Can you work these out from the model? Positions are in its coordinate system, mm. A direction names the side the tool comes from. Coordinates: 2 decimals unless noted, no trailing zeros. Order: outer loops, then holes, each group sorted by start corner. A loop starts at its lowest first (then second) coordinate and runs counter-clockwise, first axis right, second up.
```python
from build123d import *

# Parameters (mm, degrees)
SKETCH3_R          = 3
CUT_EXTRUDE1_DEPTH = 131


with BuildPart() as part:
    # Sketch2 → Revolve1 (revolve)
    with BuildSketch(Plane(origin=(0, 0, 0), x_dir=(0, 0, -1), z_dir=(1, 0, 0))):
        Polygon((0, 0), (34, 0), (34, 10), (17.5, 10), (17.5, 130), (0, 130), align=None)
    revolve(axis=Axis((0, 0, 0), (0, 1, 0)))

    # Sketch3 → Cut-Extrude1 (cut, through all)
    with BuildSketch(Plane.XZ):
        with Locations((27, 0)):
            Circle(SKETCH3_R)
        with Locations((19.091883092, -19.091883092)):
            Circle(SKETCH3_R)
        with Locations((0, -27)):
            Circle(SKETCH3_R)
        with Locations((-19.091883092, -19.091883092)):
            Circle(SKETCH3_R)
        with Locations((-27, 0)):
            Circle(SKETCH3_R)
        with Locations((-19.091883092, 19.091883092)):
            Circle(SKETCH3_R)
        with Locations((0, 27)):
            Circle(SKETCH3_R)
        with Locations((19.091883092, 19.091883092)):
            Circle(SKETCH3_R)
    extrude(amount=-CUT_EXTRUDE1_DEPTH, mode=Mode.SUBTRACT)


solid = part.part
```
1. Please list where these lines run through material, in increasing order: probe 1 along Z at (x, y) = (0, 7.75); probe 2 along Y at (x, z) = (24, -5); probe 3 along X at (y, z) = (37, -0.5).
Completed:
probe 1: z = -34 to -30, -24 to 24, 30 to 34
probe 2: y = 0 to 10
probe 3: x = -17.49 to 17.49
2. On a 3-axis mill with a long thin cutter (end or side, diameter ignored), from which of +Z, -Z, +X, -X, +Y, -Y can I reach the whole of each face in a straight line? I mean faces 1 (the cylindrical face through (10.648, 70.84, 13.887)), 2 (the cylindrical face through (18.442, 4.93, 16.163)). Say none if no direction works.
Completed:
face 1: +Y
face 2: +Y, -Y
3. Imagine slicing it at C-C on x = 27. Please give me the cut outline in (y, z).
Completed:
outline: (0, -20.66) - (10, -20.66) - (10, -3) - (0, -3) - close; (0, 3) - (10, 3) - (10, 20.66) - (0, 20.66) - close
4. Thinking about a two-plate mould opening in Z: for faces 3 (the flat face through (0, 0, 0)), 4 (the cylindrical face through (-30, 5, 0)), 5 (the cylindrical face through (-28.67, 5.07, -18.28)), which applies, pulls with the +Z half, pulls with the -Z half, needs draft (parallel to the pull), parting line crosses it, or undercut?
Completed:
face 3: needs draft
face 4: undercut
face 5: parting line crosses it
5. Imagine slicing it at D-D on z = 27. Please give me the cut outline in (x, y), then the cut area to 3 significant figures.
Completed:
outline: (-20.66, 0) - (-3, 0) - (-3, 10) - (-20.66, 10) - close; (3, 0) - (20.66, 0) - (20.66, 10) - (3, 10) - close
area: 353 mm2
6. I'm going to push flat-ended pins straight in: pin 1 (10 mm diameter, centred on y = 100.5, z = 9, fed in from -X); pin 2 (2 mm diameter, centred on y = 66, z = -6, fed in from +X); pin 3 (7 mm diameter, centred on x = -19.09, z = 19.09, fed in from +Y). Where does each tip first touch, or does it pass through?
Completed:
pin 1: stops at x = -17.04
pin 2: stops at x = 16.77
pin 3: stops at y = 10
7. Imagine slicing it at A-A on z = 0. Please give me the cut outline in (x, y).
Completed:
outline: (-34, 0) - (-30, 0) - (-30, 10) - (-34, 10) - close; (-24, 0) - (24, 0) - (24, 10) - (17.5, 10) - (17.5, 130) - (-17.5, 130) - (-17.5, 10) - (-24, 10) - close; (30, 0) - (34, 0) - (34, 10) - (30, 10) - close
8. Imagine slicing it at B-B on x = 0. Please give me the cut outline in (y, z).
Completed:
outline: (0, -34) - (10, -34) - (10, -30) - (0, -30) - close; (0, -24) - (10, -24) - (10, -17.5) - (130, -17.5) - (130, 17.5) - (10, 17.5) - (10, 24) - (0, 24) - close; (0, 30) - (10, 30) - (10, 34) - (0, 34) - close
